Here's the drawing with two shaded views (mm, measured from the low corner). I have some questions. A direction names the side the tool comes from. Round coordinates to 2 decimals unless told otherwise and drop trailing zeros. Loops run counter-clockwise (first coordinate to the right, second up) from the corner with the lowest first, then second, coordinate; pieces in that order, holes last.
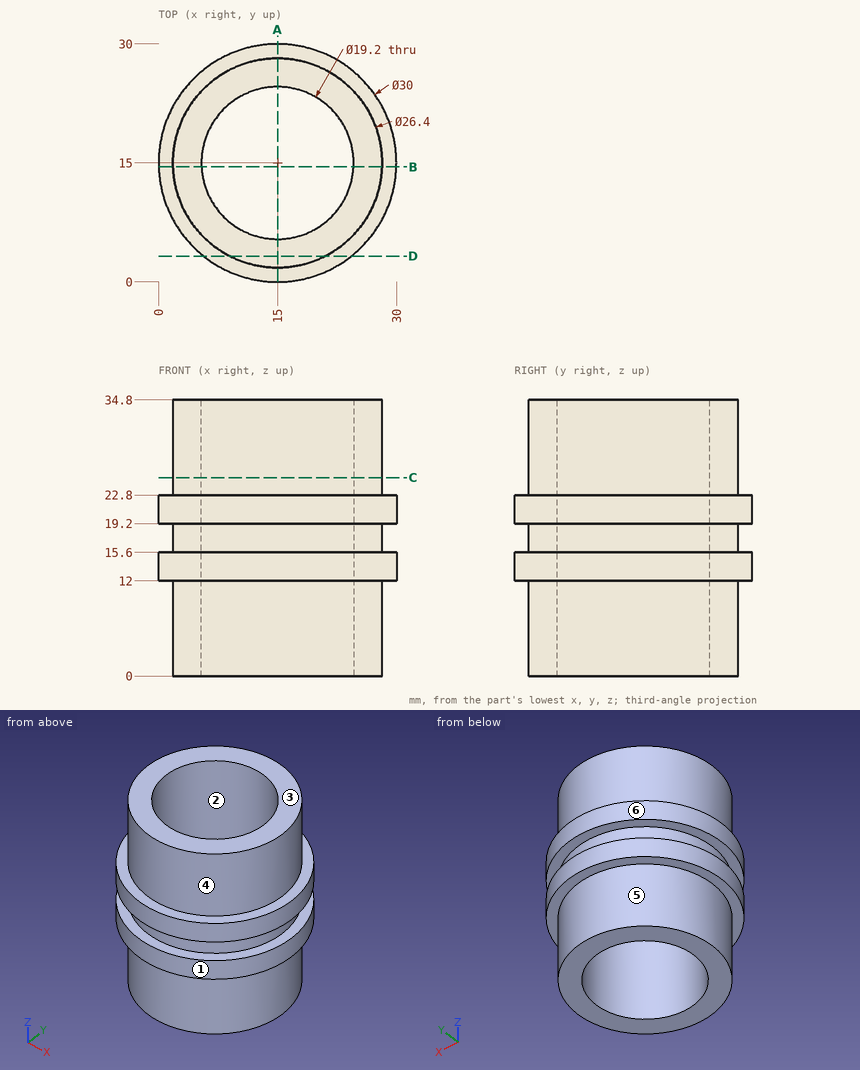
(1) Will these pins go through, and if not, where does the flat tip stop? P1, Ø1, axis at y = 7, z = 6, coming from the +X side; P2, Ø4, axis at y = 12, z = 7, coming from the +X side; P3, Ø1, axis at y = 18, z = 27, coming from the +X side.
Worked answers:
P1: stops at x = 25.86
P2: stops at x = 28.16
P3: stops at x = 27.96
(2) If we section it at D-D, the plane y = 3.25: List the corners of the cut face in (x, z) for me.
Worked answers:
outline: (5.68, 12) - (8.99, 12) - (8.99, 0) - (21.01, 0) - (21.01, 12) - (24.32, 12) - (24.32, 15.6) - (21.01, 15.6) - (21.01, 19.2) - (24.32, 19.2) - (24.32, 22.8) - (21.01, 22.8) - (21.01, 34.8) - (8.99, 34.8) - (8.99, 22.8) - (5.68, 22.8) - (5.68, 19.2) - (8.99, 19.2) - (8.99, 15.6) - (5.68, 15.6) - close
(3) If we section it at A-A, the plane x = 15: List the corners of the cut face in (y, z) for me.
Worked answers:
outline: (0, 12) - (1.8, 12) - (1.8, 0) - (5.4, 0) - (5.4, 34.8) - (1.8, 34.8) - (1.8, 22.8) - (0, 22.8) - (0, 19.2) - (1.8, 19.2) - (1.8, 15.6) - (0, 15.6) - close; (24.6, 0) - (28.2, 0) - (28.2, 12) - (30, 12) - (30, 15.6) - (28.2, 15.6) - (28.2, 19.2) - (30, 19.2) - (30, 22.8) - (28.2, 22.8) - (28.2, 34.8) - (24.6, 34.8) - close
(4) If we section it at C-C, the plane z = 25: List the corners of the cut face in (x, y) for me, then the cut area to 3 significant figures.
Worked answers:
outline: circle Ø26.4 at (15, 15); hole circle Ø19.2 at (15, 15)
area: 258 mm2
(5) For the marked faces 4, 5 and 6, which set-ups out of +Z, -Z, +X, -X, +Y, -Y let a thin tool reach every point of the face, with its end or its side?
Worked answers:
face 4: +Z
face 5: -Z
face 6: +Z, -Z
(6) If we mould it in two halves opening along Y, with no side actions, what happens to the marked faces 1, 2 and 3? For each: released by +Y, released by -Y, zero draft, split by the parting line, or undercut.
Worked answers:
face 1: split by the parting line
face 2: undercut
face 3: zero draft
(7) If I drill on line 1 (Y direction, x = 15, z = 28); line 2 (Z direction, x = 26.25, y = 22.75); line 3 (Y direction, x = 15, z = 13.5), over which ranges is the centre line in solid material (lowest first)?
Worked answers:
line 1: y = 1.8 to 5.4, 24.6 to 28.2
line 2: z = 12 to 15.6, 19.2 to 22.8
line 3: y = 0 to 5.4, 24.6 to 30
(8) If we section it at B-B, the plane y = 14.5: List the corners of the cut face in (x, z) for me, then the cut area to 3 significant figures.
Worked answers:
outline: (0.01, 12) - (1.81, 12) - (1.81, 0) - (5.41, 0) - (5.41, 34.8) - (1.81, 34.8) - (1.81, 22.8) - (0.01, 22.8) - (0.01, 19.2) - (1.81, 19.2) - (1.81, 15.6) - (0.01, 15.6) - close; (24.59, 0) - (28.19, 0) - (28.19, 12) - (29.99, 12) - (29.99, 15.6) - (28.19, 15.6) - (28.19, 19.2) - (29.99, 19.2) - (29.99, 22.8) - (28.19, 22.8) - (28.19, 34.8) - (24.59, 34.8) - close
area: 277 mm2
